Verification items for the finished model (mm, model axes). Round coordinates to 2 decimals unless told otherwise and drop trailing zeros. Loops run counter-clockwise (first coordinate to the right, second up) from the corner with the lowest first, then second, coordinate; pieces in that order, holes last. Notation, with made-up numbers: M 52.5,74.25 L 64.5,74.25 A26 ccw 64.5,103.25 Z; hole C -12.5,-3 d1. An arc over 180 degrees is marked long. Answer as CSV lines item,"result".
Autodesk Inventor part; units mm, degrees
ref_plane "YZ Plane" through (0, 0, 0) normal (1, 0, 0) x (0, 1, 0)
ref_plane "XZ Plane" through (0, 0, 0) normal (0, 1, 0) x (-1, 0, 0)
ref_plane "XY Plane" through (0, 0, 0) normal (0, 0, 1) x (1, 0, 0)
sketch "Skizze1" plane through (0, 0, 0) normal (0, 1, 0) x (-1, 0, 0)
  circle A0 centre (0, 0) radius 200
  dimension "d0" = 400
extrude "Extrusion1" add sketch "Skizze1" along normal blind 10
sketch "Skizze2" plane through (0, 10, 0) normal (0, 1, 0) x (1, 0, 0)
  circle A0 centre (0, 0) radius 200
  line L0 (0, 0) -> (200, 0) construction
  line L1 (0, 0) -> (61.8034, 190.2113)
  line L2 (0, 0) -> (200, 0) construction
  line L3 (0, 0) -> (-161.8034, 117.5571)
  line L4 (0, 0) -> (200, 0) construction
  line L5 (0, 0) -> (61.8034, -190.2113)
  line L6 (0, 0) -> (-161.8034, -117.5571)
  line L7 (0, 0) -> (200, 0)
  line L8 (200, 0) -> (100, 0)
  line L9 (0, 0) -> (30.9017, -95.1057)
  line L10 (200, 0) -> (135, 0)
  circle A1 centre (135, 0) radius 50
  line L11 (61.8034, -190.2113) -> (41.7173, -128.3926)
  circle A2 centre (41.7173, -128.3926) radius 50
  line L12 (-161.8034, -117.5571) -> (-109.2173, -79.351)
  circle A3 centre (-109.2173, -79.351) radius 50
  line L13 (-161.8034, 117.5571) -> (-109.2173, 79.351)
  circle A4 centre (-109.2173, 79.351) radius 50
  line L14 (61.8034, 190.2113) -> (41.7173, 128.3926)
  circle A5 centre (41.7173, 128.3926) radius 50
  dimension "d4" = 72
  dimension "d5" = 144
  dimension "d9" = 65
  dimension "d10" = 100
  dimension "d11" = 65
  dimension "d12" = 100
  dimension "d13" = 65
  dimension "d14" = 100
  dimension "d15" = 65
  dimension "d16" = 100
  dimension "d17" = 65
  dimension "d18" = 100
extrude "Extrusion4" cut sketch "Skizze2" against normal blind 10 contours A1 L7 | L7 A1 | A5 L1 | L1 A5 | A2 L5 | L5 A2 | A4 L3 | L3 A4 | A3 L6 | L6 A3
sketch "Skizze5" plane through (0, 0, 0) normal (0, -1, 0) x (1, 0, 0)
  circle A0 centre (0, 0) radius 22.5
  dimension "d27" = 45
extrude "Extrusion5" cut sketch "Skizze5" against normal blind 10
properties part number "Drehplatte_Rahmenvorrrichtung"
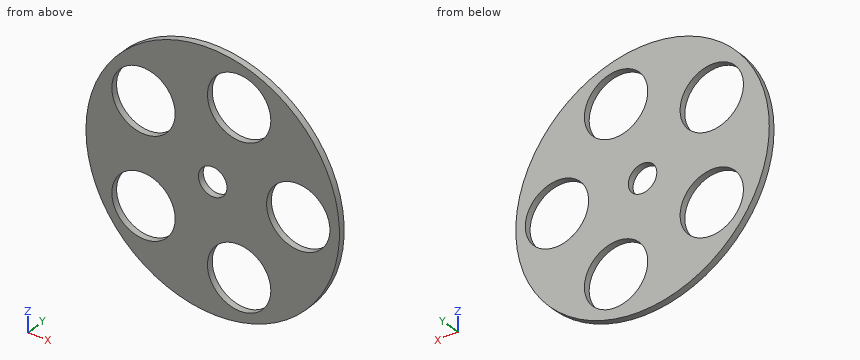
1) Go/stop test with flat-tipped pins: pin 1 (1.5 mm diameter, centred on x = -103.5, y = 5.5, fed in from +Z); pin 2 (1.5 mm diameter, centred on x = -85, y = 5.5, fed in from +Z); pin 3 (4 mm diameter, centred on y = 5, z = 66, fed in from +X). Record where each tip stops, or that it passes through.
Here are the results:
pin 1,"stops at z = 171.59"
pin 2,"stops at z = 181.39"
pin 3,"stops at x = 189.48"
2) Section check D-D (y = 2.5). Record the cut outline in (x, z).
Here are the results:
outline,"C 0,0 d400; hole C -109.22,-79.35 d100; hole C -109.22,79.35 d100; hole C 0,0 d45; hole C 41.72,-128.39 d100; hole C 41.72,128.39 d100; hole C 135,0 d100"
3) Section check B-B (z = 0). Record the cut outline in (x, y), plus the area to 3 significant figures.
Here are the results:
outline,"M -200,0 L -22.5,0 L -22.5,10 L -200,10 Z; M 22.5,0 L 85,0 L 85,10 L 22.5,10 Z; M 185,0 L 200,0 L 200,10 L 185,10 Z"
area,"2,550 mm^2"
4) Section check C-C (x = -140). Record the cut outline in (y, z), plus the area to 3 significant figures.
Here are the results:
outline,"M 0,-142.83 L 10,-142.83 L 10,-118.75 L 0,-118.75 Z; M 0,-39.95 L 10,-39.95 L 10,39.95 L 0,39.95 Z; M 0,118.75 L 10,118.75 L 10,142.83 L 0,142.83 Z"
area,"1,280 mm^2"
5) Material ranges on probe 1 along X at (y, z) = (6, 8.5); probe 2 along X at (y, z) = (6, 2.5); probe 3 along Z at (x, y) = (-67.5, 6.75), recorded low to high.
Here are the results:
probe 1,"x = -199.82 to -20.83, 20.83 to 85.73, 184.27 to 199.82"
probe 2,"x = -199.98 to -22.36, 22.36 to 85.06, 184.94 to 199.98"
probe 3,"z = -188.27 to -106.91, -51.79 to 51.79, 106.91 to 188.27"
6) Section check A-A (x = 135). Record the cut outline in (y, z).
Here are the results:
outline,"M 0,-147.56 L 10,-147.56 L 10,-50 L 0,-50 Z; M 0,50 L 10,50 L 10,147.56 L 0,147.56 Z"
